```python
from build123d import *

# Parameters (mm, degrees)
SKETCH1_W            = 120
SKETCH1_H            = 100
BOSS_EXTRUDE2_DEPTH  = 70
FILLET1_R            = 15
SHELL2_T             = -3
SKETCH3_W            = 4
SKETCH3_H            = 41
CUT_EXTRUDE1_DEPTH   = 2
SKETCH4_W            = 10
SKETCH4_H            = 70
BOSS_EXTRUDE3_DEPTH  = 2.85
SKETCH16_R           = 3.5
SKETCH16_R_2         = 2.2
SKETCH16_R_3         = 1.5
BOSS_EXTRUDE5_DEPTH  = 5
BOSS_EXTRUDE6_DEPTH  = 3
SKETCH23_R           = 3
SKETCH23_R_2         = 1.7
BOSS_EXTRUDE10_DEPTH = 4
SKETCH6_R            = 2.2
CUT_EXTRUDE2_DEPTH   = 137.014705087
SKETCH24_R           = 4
CUT_EXTRUDE3_DEPTH   = 3


with BuildPart() as part:
    # Sketch1 → Boss-Extrude2 (new body)
    with BuildSketch(Plane(origin=(0, 0, 0), x_dir=(0, 0, -1), z_dir=(1, 0, 0))):
        Rectangle(SKETCH1_W, SKETCH1_H)
    extrude(amount=BOSS_EXTRUDE2_DEPTH)

    # Fillet1
    fillet1_edges = [part.edges().sort_by_distance(p)[0] for p in [
        (35, -50, -60),
        (35, -50, 60),
        (35, 50, 60),
        (35, 50, -60),
    ]]
    fillet(fillet1_edges, radius=FILLET1_R)

    # Shell2
    shell2_openings = [part.faces().sort_by_distance(p)[0] for p in [
        (70, 0, 0),
    ]]
    offset(amount=SHELL2_T, openings=shell2_openings, kind=Kind.INTERSECTION)

    # Sketch3 → Cut-Extrude1 (cut)
    with BuildSketch(Plane.XY.offset(-57)):
        with Locations((68, 0)):
            Rectangle(SKETCH3_W, SKETCH3_H)
    extrude(amount=-CUT_EXTRUDE1_DEPTH, mode=Mode.SUBTRACT)

    # Sketch4 → Boss-Extrude3 (add)
    with BuildSketch(Plane.XY.offset(-57)):
        with Locations((25, 0)):
            Rectangle(SKETCH4_W, SKETCH4_H)
    extrude(amount=BOSS_EXTRUDE3_DEPTH)

    # Sketch16 → Boss-Extrude5 (add)
    # profile 1 of 4: a face of its own
    with BuildSketch(Plane(origin=(3, 0, 0), x_dir=(0, 0, -1), z_dir=(1, 0, 0))):
        with Locations((1.5, -29.8)):
            Circle(SKETCH16_R)
        with Locations((1.5, -29.8)):
            Circle(SKETCH16_R_2, mode=Mode.SUBTRACT)
    # profile 2 of 4: a face of its own
    with BuildSketch(Plane(origin=(3, 0, 0), x_dir=(0, 0, -1), z_dir=(1, 0, 0))):
        with Locations((-0.4, 36.2)):
            Circle(SKETCH16_R)
        with Locations((-0.4, 36.2)):
            Circle(SKETCH16_R_2, mode=Mode.SUBTRACT)
    # profile 3 of 4: a face of its own
    with BuildSketch(Plane(origin=(3, 0, 0), x_dir=(0, 0, -1), z_dir=(1, 0, 0))):
        with Locations((-38, 35)):
            Circle(SKETCH16_R_3)
    # profile 4 of 4: a face of its own
    with BuildSketch(Plane(origin=(3, 0, 0), x_dir=(0, 0, -1), z_dir=(1, 0, 0))):
        with Locations((-41.675568993, -27.374268476)):
            Circle(SKETCH16_R_3)
    extrude(amount=BOSS_EXTRUDE5_DEPTH)

    # Sketch15 → Boss-Extrude6 (add)
    with BuildSketch(Plane.XZ.offset(-47)):
        Polygon((46, -5.5), (68, -5.5), (68, -7.5), (48, -7.5), (48, -10), (68, -10), (68, -12), (46, -12), align=None)
    boss_extrude6 = extrude(amount=BOSS_EXTRUDE6_DEPTH)

    # Mirror1: Boss-Extrude6 across plane
    add(boss_extrude6.mirror(Plane.ZX))

    # Sketch23 → Boss-Extrude10 (add)
    # profile 1 of 2: a face of its own
    with BuildSketch(Plane(origin=(0, -47, 0), x_dir=(1, 0, 0), z_dir=(0, 1, 0))):
        with Locations(Location((43, -1.5, 0), (0, 0, 270))):
            Circle(SKETCH23_R)
        with Locations(Location((43, -1.5, 0), (0, 0, 270))):
            Circle(SKETCH23_R_2, mode=Mode.SUBTRACT)
    # profile 2 of 2: a face of its own
    with BuildSketch(Plane(origin=(0, -47, 0), x_dir=(1, 0, 0), z_dir=(0, 1, 0))):
        with Locations(Location((28, -32.5, 0), (0, 0, 270))):
            Circle(SKETCH23_R)
        with Locations(Location((28, -32.5, 0), (0, 0, 270))):
            Circle(SKETCH23_R_2, mode=Mode.SUBTRACT)
    extrude(amount=BOSS_EXTRUDE10_DEPTH)

    # Sketch6 → Cut-Extrude2 (cut, through all)
    with BuildSketch(Plane.XZ.offset(50)):
        with Locations(Location((65, 40, 0), (0, 0, 270))):
            Circle(SKETCH6_R)
    extrude(amount=-CUT_EXTRUDE2_DEPTH, mode=Mode.SUBTRACT)

    # Sketch24 → Cut-Extrude3 (cut)
    with BuildSketch(Plane(origin=(3, 0, 0), x_dir=(0, 0, -1), z_dir=(1, 0, 0))):
        with Locations((-10, 10)):
            Circle(SKETCH24_R)
        with Locations((10, 10)):
            Circle(SKETCH24_R)
        with Locations((-10, -10)):
            Circle(SKETCH24_R)
        with Locations((10, -10)):
            Circle(SKETCH24_R)
    extrude(amount=-CUT_EXTRUDE3_DEPTH, mode=Mode.SUBTRACT)


solid = part.part
```
Geometry check sheet. Reference: the model listing, model coordinates, mm. A direction names the side the tool comes from. Give positions to 0.01 mm unless a question says otherwise; leave off trailing zeros. Write each loop counter-clockwise with the first axis right and the second up, starting at its lowest first coordinate (ties: lowest second). Pieces come first, ordered by that corner, then holes. Notation, with made-up numbers: (17, 53.25) -> (75, 53.25) arc R24 ccw to (75, 85.25) -> close; hole circle Ø9 at (41, -1). An arc over 180 degrees is marked (long way). One line per question, with ' | ' between items.
Item 1: Sectioned sample at C-C, the plane z = -23. Record the boundary of the cut face in (x, y).
Determined:
outline: (0, -50) -> (70, -50) -> (70, -47) -> (3, -47) -> (3, 47) -> (70, 47) -> (70, 50) -> (0, 50) -> close
Item 2: Depth check by flat-ended pin: pin 1 (10 mm diameter, centred on x = 22, y = 38, fed in from -Z); pin 2 (3.5 mm diameter, centred on y = -29.5, z = -1.5, fed in from +X); pin 3 (3.5 mm diameter, centred on x = 60, y = -45.5, fed in from +Z); pin 4 (7.5 mm diameter, centred on y = 35.5, z = 1.5, fed in from +X). Enter the tip coordinate at first touch or a pass-through.
Determined:
pin 1: z = -60 | pin 2: x = 3 | pin 3: z = 57.18 | pin 4: x = 8
Item 3: Sectioned sample at B-B, the plane z = 10. Record the boundary of the cut face in (x, y).
Determined:
outline: (0, -50) -> (70, -50) -> (70, -47) -> (3, -47) -> (3, -14) -> (0, -14) -> close; (0, -6) -> (3, -6) -> (3, 6) -> (0, 6) -> close; (0, 14) -> (3, 14) -> (3, 47) -> (70, 47) -> (70, 50) -> (0, 50) -> close
Item 4: Sectioned sample at A-A, the plane x = 37. Record the boundary of the cut face in (y, z), plus the area to 3 significant figures.
Determined:
outline: (-50, -45) arc R15 ccw to (-35, -60) -> (35, -60) arc R15 ccw to (50, -45) -> (50, 45) arc R15 ccw to (35, 60) -> (-35, 60) arc R15 ccw to (-50, 45) -> close; hole (-47, -45) arc R12 ccw to (-35, -57) -> (35, -57) arc R12 ccw to (47, -45) -> (47, 45) arc R12 ccw to (35, 57) -> (-35, 57) arc R12 ccw to (-47, 45) -> close | area: 1,210 mm^2
Item 5: Scan lines: line 1 along Y through (x, z) = (1.8, 10); line 2 along X through (y, z) = (-45.5, 32.5); line 3 along Z through (x, y) = (42.5, -3). Record each from-to range of solid material in increasing order.
Determined:
line 1: -50 to -14, -6 to 6, 14 to 50 | line 2: 0 to 3, 25 to 26.3, 29.7 to 31 | line 3: -60 to -57, 57 to 60
Item 6: Sectioned sample at D-D, the plane y = -2. Record the boundary of the cut face in (x, z), plus the area to 4 significant figures.
Determined:
outline: (0, -60) -> (70, -60) -> (70, -59) -> (66, -59) -> (66, -57) -> (30, -57) -> (30, -54.15) -> (20, -54.15) -> (20, -57) -> (3, -57) -> (3, 57) -> (70, 57) -> (70, 60) -> (0, 60) -> close | area: 782.5 mm^2
Item 7: Draft check along X on faces 1 (the flat face through (11, 0, -57)), 2 (the cylindrical face through (5.46, 38.38, 0.69)), 3 (the flat face through (20, 0, -56)). Enter one of: released by +X, released by -X, zero draft, split by the parting line, or undercut.
Determined:
face 1: undercut | face 2: zero draft | face 3: undercut
Item 8: Access from +Z, -Z, +X, -X, +Y, -Y to the whole of each face (thin tool, end or side, straight path). Record for faces 4 (the flat face through (35, 0, 60)), 5 (the flat face through (36, 0, 57)), 6 (the cylindrical face through (28.1, -45, 29.5)).
Determined:
face 4: +Z, +X, -X, +Y, -Y | face 5: +X | face 6: none
